from build123d import *

# Parameters (mm, degrees)
SKETCH2_R           = 2.25
BOSS_EXTRUDE1_DEPTH = 4.7625


with BuildPart() as part:
    # Sketch2 → Boss-Extrude1 (new body)
    with BuildSketch(Plane.XY):
        with BuildLine():
            Line((-68.055152616, 8.002600295), (-68.055152616, -49.587169128))
            ThreePointArc((-68.055152616, -49.587169128), (-68.738717517, -53.22090509), (-70.695960025, -56.35786218))
            ThreePointArc((-70.695960025, -56.35786218), (-70.531296713, -64.268428513), (-62.62073038, -64.433091825))
            ThreePointArc((-62.62073038, -64.433091825), (-59.48377329, -62.475849317), (-55.850037328, -61.792284416))
            Line((-55.850037328, -61.792284416), (37.739732095, -61.792284416))
            ThreePointArc((37.739732095, -61.792284416), (41.373468058, -62.475849317), (44.510425147, -64.433091825))
            ThreePointArc((44.510425147, -64.433091825), (52.420991481, -64.268428513), (52.585654792, -56.35786218))
            ThreePointArc((52.585654792, -56.35786218), (50.628412285, -53.22090509), (49.944847384, -49.587169128))
            Line((49.944847384, -49.587169128), (49.944847384, 8.002600295))
            ThreePointArc((49.944847384, 8.002600295), (50.628412285, 11.636336257), (52.585654792, 14.773293347))
            ThreePointArc((52.585654792, 14.773293347), (52.420991481, 22.683859681), (44.510425147, 22.848522992))
            ThreePointArc((44.510425147, 22.848522992), (41.373468058, 20.891280484), (37.739732095, 20.207715584))
            Line((37.739732095, 20.207715584), (-55.850037328, 20.207715584))
            ThreePointArc((-55.850037328, 20.207715584), (-59.48377329, 20.891280484), (-62.62073038, 22.848522992))
            ThreePointArc((-62.62073038, 22.848522992), (-70.531296713, 22.683859681), (-70.695960025, 14.773293347))
            ThreePointArc((-70.695960025, 14.773293347), (-68.738717517, 11.636336257), (-68.055152616, 8.002600295))
        make_face()
        with Locations(Location((-66.490181459, 18.642744426, 0), (0, 0, 180))):
            Circle(SKETCH2_R, mode=Mode.SUBTRACT)
        with Locations(Location((48.379876226, 18.642744426, 0), (0, 0, 180))):
            Circle(SKETCH2_R, mode=Mode.SUBTRACT)
        with Locations(Location((48.379876226, -60.227313259, 0), (0, 0, 180))):
            Circle(SKETCH2_R, mode=Mode.SUBTRACT)
        with Locations(Location((-66.490181459, -60.227313259, 0), (0, 0, 180))):
            Circle(SKETCH2_R, mode=Mode.SUBTRACT)
        with BuildLine():
            Line((30.076846635, 0.887717024), (18.876846635, 0.88771689))
            ThreePointArc((18.876846635, 0.88771689), (14.404396266, -0.964832772), (12.551846711, -5.437283185))
            Line((12.551846711, -5.437283185), (12.55184708, -36.437283185))
            ThreePointArc((12.55184708, -36.437283185), (14.404396743, -40.909733554), (18.876847156, -42.76228311))
            Line((18.876847156, -42.76228311), (30.076847156, -42.762282976))
            ThreePointArc((30.076847156, -42.762282976), (34.549297525, -40.909733314), (36.40184708, -36.437282901))
            Line((36.40184708, -36.437282901), (36.401846949, -25.437282901))
            Line((36.401846949, -25.437282901), (38.276846863, -25.437282901))
            Line((38.276846863, -25.437282901), (38.276846863, -23.637282901))
            Line((38.276846863, -23.637282901), (36.401846928, -23.637282901))
            Line((36.401846928, -23.637282901), (36.401846863, -18.237282901))
            Line((36.401846863, -18.237282901), (38.276846863, -18.237282879))
            Line((38.276846863, -18.237282879), (38.276846842, -16.437282879))
            Line((38.276846842, -16.437282879), (36.401846842, -16.437282901))
            Line((36.401846842, -16.437282901), (36.401846711, -5.437282901))
            ThreePointArc((36.401846711, -5.437282901), (34.549297048, -0.964832532), (30.076846635, 0.887717024))
        make_face(mode=Mode.SUBTRACT)
    extrude(amount=BOSS_EXTRUDE1_DEPTH)


solid = part.part
Verification items for the finished model (mm, model axes). A direction names the side the tool comes from. Coordinates: 2 decimals unless noted, no trailing zeros. Write each loop counter-clockwise with the first axis right and the second up, starting at its lowest first coordinate (ties: lowest second). Pieces come first, ordered by that corner, then holes. Notation, with made-up numbers: M 81,-23.75 L 89,-23.75 A16 cw 89,-7.75 Z; hole C -28,-6 d2. An arc over 180 degrees is marked long. Use CSV: the item, a comma, the result in double quotes.
Q1. Thickness scan on line 1 along Y through (x, z) = (48.5, 3); line 2 along X through (y, z) = (-37, 3.8); line 3 along Y through (x, z) = (-65.5, 0.7). Record the ranges inside material, lowest first. Write a range as [from, to].
Computed values:
line 1,"[-65.94, -62.47], [-57.98, 16.4], [20.89, 24.36]"
line 2,"[-68.06, 12.58], [36.38, 49.94]"
line 3,"[-65.86, -62.25], [-58.21, 16.62], [20.66, 24.27]"
Q2. Section check C-C, the plane y = 6. Enter the section's corners in (x, z).
Computed values:
outline,"M -68.06,0 L 49.94,0 L 49.94,4.76 L -68.06,4.76 Z"
Q3. Mould release check, pull along Y, two halves, no side actions. Record for faces 6 (the flat face through (-10, -20, 4.762)), 7 (the cylindrical face through (14.45, -0.92, 2.35)), 8 (the cylindrical face through (34.5, -40.96, 2.35)), 9 (the cylindrical face through (41.4, 20.9, 2.3)): pulls with the +Y half, pulls with the -Y half, needs draft (parallel to the pull), parting line crosses it, or undercut.
Computed values:
face 6,"needs draft"
face 7,"undercut"
face 8,"undercut"
face 9,"pulls with the +Y half"
Q4. Set-up check for faces 1 (the flat face through (-10, -61.792, 2)), 2 (the cylindrical face through (-68.72, -53.17, 2.35)), 3 (the cylindrical face through (50.647, -53.269, 2.348)), 4 (the flat face through (25, 0.888, 2)), 5 (the flat face through (-8, 20.208, 2)): record each of +Z, -Z, +X, -X, +Y, -Y from which the full face is reachable in a straight line by a thin tool's end or side.
Computed values:
face 1,"+Z, -Z, -Y"
face 2,"+Z, -Z, -X"
face 3,"+Z, -Z, +X"
face 4,"+Z, -Z"
face 5,"+Z, -Z, +Y"
Q5. Section check D-D, the plane z = 1.8. State how many separate pieces and enclosed holes the cut face has, and give its area (3 significant figures).
Computed values:
separate pieces,"1"
enclosed holes,"5"
area,"8,850 mm²"
Q6. Section check B-B, the plane x = -1.5. Enter the section's corners in (y, z).
Computed values:
outline,"M -61.79,0 L 20.21,0 L 20.21,4.76 L -61.79,4.76 Z"
Q7. Section check A-A, the plane y = -30.5. Enter the section's corners in (x, z), and give its area (3 significant figures).
Computed values:
outline,"M -68.06,0 L 12.55,0 L 12.55,4.76 L -68.06,4.76 Z; M 36.4,0 L 49.94,0 L 49.94,4.76 L 36.4,4.76 Z"
area,"448 mm²"
Q8. Go/stop test with flat-tipped pins: P1, Ø1.4, axis at y = -21, z = 2.5, coming from the -X side; P2, Ø0.6, axis at x = 37.5, z = 1.5, coming from the -Y side; P3, Ø1.5, axis at x = 37.5, z = 2, coming from the +Y side. Record where each tip stops, or that it passes through.
Computed values:
P1,"x = -68.06"
P2,"y = -61.79"
P3,"y = 20.22"
